Design review of the part built by this model. Coordinates are the model's own, in mm. Give positions to 0.01 mm unless a question says otherwise; leave off trailing zeros. Order: outer loops, then holes, each group sorted by start corner. A loop starts at its lowest first (then second) coordinate and runs counter-clockwise, first axis right, second up. Notation, with made-up numbers: M -7.5,5 L -2.5,5 A24 ccw -2.5,44 Z; hole C 19,66 d7. An arc over 180 degrees is marked long. Put each result on its own line as item: value. Start each with the question number.
from build123d import *

# Parameters (mm, degrees)
BOSS_EXTRUDE1_DEPTH             = 2.286
TAP_DRILL_FOR_M3X0_5_TAP1_D     = 2.5
TAP_DRILL_FOR_M3X0_5_TAP1_DEPTH = 25.4
TAP_DRILL_FOR_M3X0_5_TAP1_TIP   = 0.751075774


with BuildPart() as part:
    # Sketch1 → Boss-Extrude1 (new body)
    with BuildSketch(Plane.YZ):
        Polygon((0, -3.15290982), (2.7305, -1.57645491), (2.7305, 1.57645491), (0, 3.15290982), (-2.7305, 1.57645491), (-2.7305, -1.57645491), align=None)
    extrude(amount=BOSS_EXTRUDE1_DEPTH)

    # Tap Drill for M3x0.5 Tap1
    with Locations(Plane(origin=(2.286, 0, 0), x_dir=(0, 0, -1), z_dir=(1, 0, 0))):
        with Locations((0, 0)):
            Hole(TAP_DRILL_FOR_M3X0_5_TAP1_D / 2, depth=TAP_DRILL_FOR_M3X0_5_TAP1_DEPTH)
            with Locations((0, 0, -(TAP_DRILL_FOR_M3X0_5_TAP1_DEPTH + TAP_DRILL_FOR_M3X0_5_TAP1_TIP / 2))):  # 118° drill point
                Cone(0, TAP_DRILL_FOR_M3X0_5_TAP1_D / 2, TAP_DRILL_FOR_M3X0_5_TAP1_TIP, mode=Mode.SUBTRACT)


solid = part.part
1. To check wall thickness, follow probe 1 along Y at (x, z) = (0.7, 0); probe 2 along Y at (x, z) = (1.2, -1); probe 3 along Z at (x, y) = (0.35, 0.9). State the ranges of each line that lie inside material, in increasing order.
2. Insertion check: pin 1 (1 mm diameter, centred on x = 0.5, y = -1.5, fed in from -Z). The pin has a flat end and moves straight along its axis. Give the tip position at first contact, or say it passes through.
3. Consider section B-B on x = 1.6. Give the boundary of the cut face in (y, z).
4. The part is to be moulded in two halves that separate along Z. For faces 1 (the flat face through (1.127, 1.384, 2.354)), 2 (the flat face through (1.127, -1.384, -2.354)), 3 (the cylindrical face through (1.13, -1.22, -0.27)), say which applies: +Z half, -Z half, draft (parallel to the pull), parting line (faces both ways), or undercut.
5. Consider section D-D on y = -2.4. Give the boundary of the cut face in (x, z).
6. Consider section A-A on z = 0. Give the boundary of the cut face in (x, y), then the cut area to 3 significant figures.
7. Consider section C-C on y = 0.3. Give the boundary of the cut face in (x, z).
Returned:
1. probe 1: y = -2.73 to -1.25, 1.25 to 2.73
1. probe 2: y = -2.73 to -0.75, 0.75 to 2.73
1. probe 3: z = -2.63 to -0.87, 0.87 to 2.63
2. pin 1: stops at z = -2.58
3. outline: M -2.73,-1.58 L 0,-3.15 L 2.73,-1.58 L 2.73,1.58 L 0,3.15 L -2.73,1.58 Z; hole C 0,0 d2.5
4. face 1: +Z half
4. face 2: -Z half
4. face 3: undercut
5. outline: M 0,-1.77 L 2.29,-1.77 L 2.29,1.77 L 0,1.77 Z
6. outline: M 0,-2.73 L 2.29,-2.73 L 2.29,-1.25 L 0,-1.25 Z; M 0,1.25 L 2.29,1.25 L 2.29,2.73 L 0,2.73 Z
6. area: 6.77 mm2
7. outline: M 0,-2.98 L 2.29,-2.98 L 2.29,-1.21 L 0,-1.21 Z; M 0,1.21 L 2.29,1.21 L 2.29,2.98 L 0,2.98 Z
